Could you check a few things on this model? Use its own coordinates, in mm. A direction names the side the tool comes from. Give positions to 0.01 mm unless a question says otherwise; leave off trailing zeros. Write each loop counter-clockwise with the first axis right and the second up, starting at its lowest first coordinate (ties: lowest second). Pieces come first, ordered by that corner, then holes. Notation, with made-up numbers: M 46,51.25 L 90,51.25 A31 cw 90,78.25 Z; hole C 34.25,26 d7. An arc over 180 degrees is marked long. Answer as CSV lines item,"result". Start each with the question number.
from build123d import *

# Parameters (mm, degrees)
ESQUISSE1_R             = 32.5
BOSS_EXTRU_1_DEPTH      = 4
ESQUISSE2_R             = 32.5
ESQUISSE2_R_2           = 25
BOSS_EXTRU_2_DEPTH      = 6
ESQUISSE3_R             = 1.5
ENL_V_MAT_EXTRU_1_DEPTH = 11
ESQUISSE4_R             = 12.5
ENL_V_MAT_EXTRU_2_DEPTH = 6


with BuildPart() as part:
    # Esquisse1 → Boss.-Extru.1 (new body)
    with BuildSketch(Plane.XY):
        Circle(ESQUISSE1_R)
    extrude(amount=BOSS_EXTRU_1_DEPTH)

    # Esquisse2 → Boss.-Extru.2 (add)
    with BuildSketch(Plane.XY.offset(4)):
        Circle(ESQUISSE2_R)
        Circle(ESQUISSE2_R_2, mode=Mode.SUBTRACT)
    extrude(amount=BOSS_EXTRU_2_DEPTH)

    # Esquisse3 → Enlèv. mat.-Extru.1 (cut, through all)
    with BuildSketch(Plane.XY.offset(10)):
        with Locations((0, 28.75)):
            Circle(ESQUISSE3_R)
        with Locations((28.75, 0)):
            Circle(ESQUISSE3_R)
        with Locations((0, -28.75)):
            Circle(ESQUISSE3_R)
        with Locations((-28.75, 0)):
            Circle(ESQUISSE3_R)
    extrude(amount=-ENL_V_MAT_EXTRU_1_DEPTH, mode=Mode.SUBTRACT)

    # Esquisse4 → Enlèv. mat.-Extru.2 (cut)
    with BuildSketch(Plane(origin=(0, 0, 0), x_dir=(-1, 0, 0), z_dir=(0, 0, -1))):
        Circle(ESQUISSE4_R)
    extrude(amount=-ENL_V_MAT_EXTRU_2_DEPTH, mode=Mode.SUBTRACT)


solid = part.part
1. Thinking about a two-plate mould opening in Y: for faces 3 (the flat face through (17, -19, 10)), 4 (the cylindrical face through (-0.195, 30.237, 5.07)), 5 (the cylindrical face through (31, 9.76, 4.93)), which applies, pulls with the +Y half, pulls with the -Y half, needs draft (parallel to the pull), parting line crosses it, or undercut?
2. Imagine slicing it at A-A, the plane x = 0. Please give me the cut outline in (y, z), plus the area to 3 significant figures.
3. Please list where these lines run through material, in increasing order: line 1 (Y direction, x = 0, z = 7.95); line 2 (X direction, y = 0.5, z = 1.25); line 3 (Y direction, x = 17, z = 7.75).
4. Imagine slicing it at B-B, the plane x = -28.75. Please give me the cut outline in (y, z).
5. Will these pins go through, and if not, where does the flat tip stop? P1, Ø1.5, axis at y = 18, z = 3.5, coming from the +X side; P2, Ø1.5, axis at y = -9.5, z = 1, coming from the -X side; P3, Ø15, axis at x = 6, y = -6.5, coming from the +Z side.
6. On a 3-axis mill with a long thin cutter (end or side, diameter ignored), from which of +Z, -Z, +X, -X, +Y, -Y can I reach the whole of each face in a straight line? I mean faces 1 (the cylindrical face through (27.25, 0.07, 5.07)), 2 (the cylindrical face through (23.846, 7.509, 6.958)). Say none if no direction works.
7. Imagine slicing it at C-C, the plane z = 8. Please give me the cut outline in (x, y), plus the area to 3 significant figures.
Solutions:
1,face 3,"needs draft"
1,face 4,"undercut"
1,face 5,"parting line crosses it"
2,outline,"M -32.5,0 L -30.25,0 L -30.25,10 L -32.5,10 Z; M -27.25,0 L -12.5,0 L -12.5,4 L -25,4 L -25,10 L -27.25,10 Z; M 12.5,0 L 27.25,0 L 27.25,10 L 25,10 L 25,4 L 12.5,4 Z; M 30.25,0 L 32.5,0 L 32.5,10 L 30.25,10 Z"
2,area,"190 mm²"
3,line 1,"-32.5 to -30.25, -27.25 to -25, 25 to 27.25, 30.25 to 32.5"
3,line 2,"-32.5 to -30.16, -27.34 to -12.49, 12.49 to 27.34, 30.16 to 32.5"
3,line 3,"-27.7 to -18.33, 18.33 to 27.7"
4,outline,"M -15.16,0 L -1.5,0 L -1.5,10 L -15.16,10 Z; M 1.5,0 L 15.16,0 L 15.16,10 L 1.5,10 Z"
5,P1,"x = 27.54"
5,P2,"x = -31.3"
5,P3,"z = 4"
6,face 1,"+Z, -Z"
6,face 2,"+Z"
7,outline,"C 0,0 d65; hole C -28.75,0 d3; hole C 0,0 d50; hole C 0,-28.75 d3; hole C 0,28.75 d3; hole C 28.75,0 d3"
7,area,"1,330 mm²"
